```python
from build123d import *

# Parameters (mm, degrees)
SKETCH_1_W          = 43.5
SKETCH_1_H          = 43.5
EXTRUDE_1_DEPTH     = 1
SKETCH_2_R          = 1.5
CUT_EXTRUDE_1_DEPTH = 31.775396017
SKETCH_2_3_W        = 23
SKETCH_2_3_H        = 16
EXTRUDE_2_DEPTH     = 25
SKETCH_2_4_W        = 7.7
SKETCH_2_4_H        = 10
SKETCH_2_4_W_2      = 15
SKETCH_2_4_H_2      = 7.7
EXTRUDE_3_DEPTH     = 10
EXTRUDE_4_DEPTH     = 9
SKETCH_2_6_R        = 4
EXTRUDE_5_DEPTH     = 11


with BuildPart() as part:
    # Sketch 1 → Extrude 1 (new body)
    with BuildSketch(Plane(origin=(0, 0, 0), x_dir=(1, 0, 0), z_dir=(0, 1, 0))):
        Rectangle(SKETCH_1_W, SKETCH_1_H)
    extrude(amount=EXTRUDE_1_DEPTH)

    # Sketch 2 → Cut-Extrude 1 (cut, through all)
    with BuildSketch(Plane(origin=(0, 1, 0), x_dir=(1, 0, 0), z_dir=(0, 1, 0))):
        with Locations(Location((-18.25, 18.25, 0), (0, 0, 270))):
            Circle(SKETCH_2_R)
        with Locations(Location((18.25, 18.25, 0), (0, 0, 270))):
            Circle(SKETCH_2_R)
        with Locations(Location((18.25, -18.25, 0), (0, 0, 270))):
            Circle(SKETCH_2_R)
        with Locations(Location((-18.25, -18.25, 0), (0, 0, 270))):
            Circle(SKETCH_2_R)
    extrude(amount=-CUT_EXTRUDE_1_DEPTH, mode=Mode.SUBTRACT)

    # Sketch 2_3 → Extrude 2 (add)
    with BuildSketch(Plane(origin=(0, 1, 0), x_dir=(1, 0, 0), z_dir=(0, 1, 0))):
        with Locations((0, 13.75)):
            Rectangle(SKETCH_2_3_W, SKETCH_2_3_H)
    extrude(amount=EXTRUDE_2_DEPTH)

    # Sketch 2_4 → Extrude 3 (add)
    with BuildSketch(Plane(origin=(0, 1, 0), x_dir=(1, 0, 0), z_dir=(0, 1, 0))):
        with Locations((-17.9, -6.75)):
            Rectangle(SKETCH_2_4_W, SKETCH_2_4_H)
        with Locations((17.9, -6.75)):
            Rectangle(SKETCH_2_4_W, SKETCH_2_4_H)
        with Locations((-7.75, -17.9)):
            Rectangle(SKETCH_2_4_W_2, SKETCH_2_4_H_2)
    extrude(amount=EXTRUDE_3_DEPTH)

    # Sketch 2_5 → Extrude 4 (add)
    with BuildSketch(Plane(origin=(0, 1, 0), x_dir=(1, 0, 0), z_dir=(0, 1, 0))):
        Polygon((15.75, -20.75), (0.75, -20.75), (0.75, -15.75), (3.25, -15.75), (3.25, -18.25), (13.25, -18.25), (13.25, -15.75), (15.75, -15.75), align=None)
    extrude(amount=EXTRUDE_4_DEPTH)

    # Sketch 2_6 → Extrude 5 (add)
    with BuildSketch(Plane(origin=(0, 1, 0), x_dir=(1, 0, 0), z_dir=(0, 1, 0))):
        with Locations(Location((-6.75, -4.75, 0), (0, 0, 270))):
            Circle(SKETCH_2_6_R)
        with Locations(Location((7.25, -11.75, 0), (0, 0, 270))):
            Circle(SKETCH_2_6_R)
    extrude(amount=EXTRUDE_5_DEPTH)


solid = part.part
```
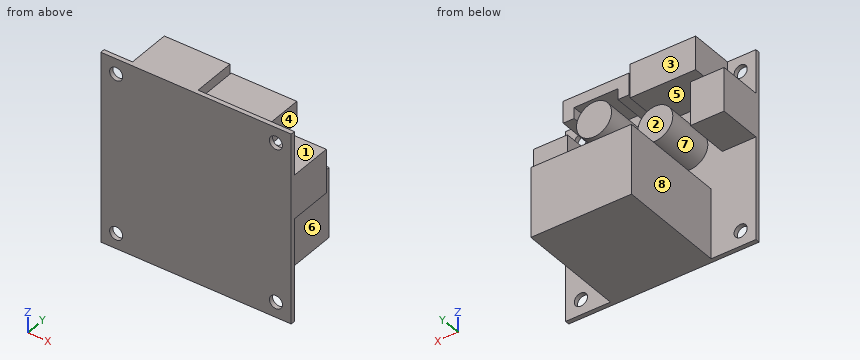
Work out the finished part from the listing and answer in its coordinate system (mm). Face numbers are marked on the shaded views. A direction names the side the tool comes from. Give positions to 0.01 mm unless a question says otherwise; leave off trailing zeros. Loops run counter-clockwise (first coordinate to the right, second up) from the corner with the lowest first, then second, coordinate; pieces in that order, holes last. Notation, with made-up numbers: (89, 24) -> (123, 24) arc R18 ccw to (123, 48) -> close; hole circle Ø8 at (0, 42). An arc over 180 degrees is marked (long way). Use CSV: the item, a comma, the result in double quotes.
1. The part is cut by section B-B (z = 4.75). Write down the section's boundary in (x, y), then the cut area to 4 significant figures.
Found:
outline,"(-21.75, 0) -> (21.75, 0) -> (21.75, 11) -> (14.05, 11) -> (14.05, 1) -> (-2.75, 1) -> (-2.75, 12) -> (-10.75, 12) -> (-10.75, 1) -> (-14.05, 1) -> (-14.05, 11) -> (-21.75, 11) -> close"
area,"285.5 mm^2"
2. The part is cut by section C-C (x = 18.25). Write down the section's boundary in (y, z), then the cut area to 4 significant figures.
Found:
outline,"(0, -21.75) -> (1, -21.75) -> (1, -19.75) -> (0, -19.75) -> close; (0, -16.75) -> (1, -16.75) -> (1, 1.75) -> (11, 1.75) -> (11, 11.75) -> (1, 11.75) -> (1, 16.75) -> (0, 16.75) -> close; (0, 19.75) -> (1, 19.75) -> (1, 21.75) -> (0, 21.75) -> close"
area,"137.5 mm^2"
3. A tool of negligible diameter and unlimited length cuts with its end or side. For the marked faces 1, 2, 3, 4 and 5, from which of +Z, -Z, +X, -X, +Y, -Y can it reach the whole face along a straight path? Write none if from no direction.
Found:
face 1,"+X, +Y"
face 2,"+Z, +X, -X, +Y"
face 3,"+Z, -X, +Y"
face 4,"+Z, +X, +Y"
face 5,"-X, +Y"
4. The mould has two halves that part along X. Classify the marked faces 6, 7 and 8: +X half, -X half, draft (parallel to the pull), parting line (faces both ways), or undercut.
Found:
face 6,"+X half"
face 7,"undercut"
face 8,"-X half"
5. Flat-ended cylindrical pins translate along their axes: pin 1 Ø2 at (x, z) = (-3, 8) entering from +Y; pin 2 Ø4 at (x, z) = (20, 4.5) entering from +Y; pin 3 Ø12 at (y, z) = (11.5, -7.5) entering from +X. Find the tip coordinate at first contact, or state that the pin passes through.
Found:
pin 1,"y = 12"
pin 2,"y = 11"
pin 3,"x = 11.5"
6. The part is cut by section A-A (y = 9.25). Write down the section's boundary in (x, z), then the cut area to 3 significant figures.
Found:
outline,"(-21.75, 1.75) -> (-14.05, 1.75) -> (-14.05, 11.75) -> (-21.75, 11.75) -> close; (-15.25, 14.05) -> (-0.25, 14.05) -> (-0.25, 21.75) -> (-15.25, 21.75) -> close; (-11.5, -21.75) -> (11.5, -21.75) -> (11.5, -5.75) -> (-11.5, -5.75) -> close; circle Ø8 at (-6.75, 4.75); (0.75, 15.75) -> (3.25, 15.75) -> (3.25, 18.25) -> (13.25, 18.25) -> (13.25, 15.75) -> (15.75, 15.75) -> (15.75, 20.75) -> (0.75, 20.75) -> close; circle Ø8 at (7.25, 11.75); (14.05, 1.75) -> (21.75, 1.75) -> (21.75, 11.75) -> (14.05, 11.75) -> close"
area,"788 mm^2"
7. Straight lines are drawn through the part: line 1 (X direction, y = 0.6, z = 18.25); line 2 (Z direction, x = -2.5, y = 6); line 3 (X direction, y = 10.75, z = 5.5). For each, find the intervals that lie inside material, in ascending order.
Found:
line 1,"-21.75 to -19.75, -16.75 to 16.75, 19.75 to 21.75"
line 2,"-21.75 to -5.75, 14.05 to 21.75"
line 3,"-21.75 to -14.05, -10.68 to -2.82, 14.05 to 21.75"
8. The part is cut by section D-D (z = 19). Write down the section's boundary in (x, y).
Found:
outline,"(-21.75, 0) -> (-19.55, 0) -> (-19.55, 1) -> (-21.75, 1) -> close; (-16.95, 0) -> (16.95, 0) -> (16.95, 1) -> (15.75, 1) -> (15.75, 10) -> (0.75, 10) -> (0.75, 1) -> (-0.25, 1) -> (-0.25, 11) -> (-15.25, 11) -> (-15.25, 1) -> (-16.95, 1) -> close; (19.55, 0) -> (21.75, 0) -> (21.75, 1) -> (19.55, 1) -> close"
